Geometry: final body of the model. Coordinates: model frame, mm. Give positions to 0.01 mm unless a question says otherwise; leave off trailing zeros. Loops run counter-clockwise (first coordinate to the right, second up) from the corner with the lowest first, then second, coordinate; pieces in that order, holes last. Notation, with made-up numbers: (85, 43) - (91, 43) arc R26 cw to (91, 72) - close; hole circle Ø1 at (24, 60.25). An arc over 180 degrees is marked (long way). Use CSV: the item, a comma, the result in double quotes. Start each with the question number.
```python
from build123d import *

# Parameters (mm, degrees)
F0_R     = 2.2
F0_R_2   = 2.7
F1_DEPTH = 5


with BuildPart() as f1:
    # F0 (on Front) → F1 (new body)
    with BuildSketch(Plane.XZ):
        with BuildLine():
            Line((-10, 0), (-10, -45))
            Line((-10, -45), (10, -45))
            Line((10, -45), (10, 0))
            ThreePointArc((10, 0), (0, 10), (-10, 0))
        make_face()
        with Locations((0, -40)):
            Circle(F0_R, mode=Mode.SUBTRACT)
        with Locations((0, -25)):
            Circle(F0_R, mode=Mode.SUBTRACT)
        Circle(F0_R_2, mode=Mode.SUBTRACT)
    extrude(amount=F1_DEPTH)


solid = f1.part
```
Item 1: Section D-D (x = 4). Output: boundary loops of the cut face in (y, z), plus the area to 3 significant figures.
Item 2: Section B-B (z = -25). Output: boundary loops of the cut face in (x, y), plus the area to 3 significant figures.
Item 3: Section C-C (x = 0.25). Output: boundary loops of the cut face in (y, z), plus the area to 3 significant figures.
Item 4: Mould query, pull axis Z, two halves, no side actions, for faces 1 (the cylindrical face through (0, -2, 10)), 2 (the flat face through (0, -2, -45)), 3 (the flat face through (0, -5, -17)), 4 (the cylindrical face through (-0.477, -2.465, -27.148)). Classes: pulls with the +Z half, pulls with the -Z half, needs draft (parallel to the pull), parting line crosses it, or undercut.
Item 5: Section A-A (y = -2.05). Output: boundary loops of the cut face in (x, z).
Item 6: Ray query, probe 1 along Z at (x, y) = (0, -1.7); probe 2 along Z at (x, y) = (-1.25, -4.3); probe 3 along X at (y, z) = (-1.4, -23). Return the intervals inside material, ascending.
Outcome:
1,outline,"(-5, -45) - (0, -45) - (0, 9.17) - (-5, 9.17) - close"
1,area,"271 mm2"
2,outline,"(-10, -5) - (-2.2, -5) - (-2.2, 0) - (-10, 0) - close; (2.2, -5) - (10, -5) - (10, 0) - (2.2, 0) - close"
2,area,"78.0 mm2"
3,outline,"(-5, -45) - (0, -45) - (0, -42.19) - (-5, -42.19) - close; (-5, -37.81) - (0, -37.81) - (0, -27.19) - (-5, -27.19) - close; (-5, -22.81) - (0, -22.81) - (0, -2.69) - (-5, -2.69) - close; (-5, 2.69) - (0, 2.69) - (0, 10) - (-5, 10) - close"
3,area,"204 mm2"
4,face 1,"pulls with the +Z half"
4,face 2,"pulls with the -Z half"
4,face 3,"needs draft"
4,face 4,"undercut"
5,outline,"(-10, -45) - (10, -45) - (10, 0) arc R10 ccw to (-10, 0) - close; hole circle Ø5.4 at (0, 0); hole circle Ø4.4 at (0, -40); hole circle Ø4.4 at (0, -25)"
6,probe 1,"z = -45 to -42.2, -37.8 to -27.2, -22.8 to -2.7, 2.7 to 10"
6,probe 2,"z = -45 to -41.81, -38.19 to -26.81, -23.19 to -2.39, 2.39 to 9.92"
6,probe 3,"x = -10 to -0.92, 0.92 to 10"
